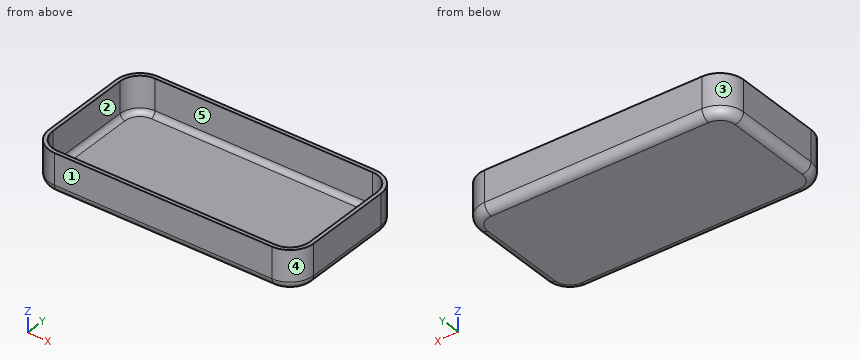
from build123d import *

# Parameters (mm, degrees)
F0_W     = 53.3
F0_H     = 27.3
F0_W_2   = 51.8
F0_H_2   = 25.8
F1_DEPTH = 0.75
F2_DEPTH = 8
F3_R     = 4
F4_R     = 4.75
F5_R     = 1
F6_R     = 1.75


with BuildPart() as f1:
    # F0 (on Top) → F1 (new body)
    with BuildSketch(Plane.XY):
        Rectangle(F0_W, F0_H)
        Rectangle(F0_W_2, F0_H_2, mode=Mode.SUBTRACT)
        Rectangle(F0_W_2, F0_H_2)
    extrude(amount=F1_DEPTH)

    # F0 (on Top) → F2 (join)
    with BuildSketch(Plane.XY):
        Rectangle(F0_W, F0_H)
        Rectangle(F0_W_2, F0_H_2, mode=Mode.SUBTRACT)
    extrude(amount=F2_DEPTH)

    # F3
    f3_edges = [f1.edges().sort_by_distance(p)[0] for p in [
        (-25.9, 12.9, 4.375),
        (25.9, 12.9, 4.375),
        (25.9, -12.9, 4.375),
        (-25.9, -12.9, 4.375),
    ]]
    fillet(f3_edges, radius=F3_R)

    # F4
    f4_edges = [f1.edges().sort_by_distance(p)[0] for p in [
        (26.65, 13.65, 4),
        (26.65, -13.65, 4),
        (-26.65, 13.65, 4),
        (-26.65, -13.65, 4),
    ]]
    fillet(f4_edges, radius=F4_R)

    # F5
    f5_edges = [f1.edges().sort_by_distance(p)[0] for p in [
        (0, 12.9, 0.75),
    ]]
    fillet(f5_edges, radius=F5_R)

    # F6
    f6_edges = [f1.edges().sort_by_distance(p)[0] for p in [
        (0, 13.65, 0),
    ]]
    fillet(f6_edges, radius=F6_R)


solid = f1.part
Can you work these out from the model? Positions are in its coordinate system, mm. Face numbers are marked on the shaded views. A direction names the side the tool comes from. Coordinates: 2 decimals unless noted, no trailing zeros. Loops run counter-clockwise (first coordinate to the right, second up) from the corner with the lowest first, then second, coordinate; pieces in that order, holes last. Notation, with made-up numbers: (81.25, 31) - (108.25, 31) arc R19 ccw to (108.25, 43) - close; hole circle Ø10 at (26, 84.25). An arc over 180 degrees is marked (long way). Answer as a JSON object with one key per item and string values. Group by question number.
Item 1: If we section it at B-B (y = -1.25): List the corners of the cut face in (x, z) for me, plus the area to 3 significant figures.
Item 2: If we section it at A-A (z = 5): List the corners of the cut face in (x, y) for me, plus the area to 3 significant figures.
Item 3: For pin 1 (1 mm diameter, centred on x = -6.5, y = -11, fed in from +Z), with a flat end and sliding along its axis, tell me the tip position at first contact or that it passes through.
Item 4: If we mould it in two halves opening along Y, with no side actions, what happens to the marked faces 3, 4 and 5? For each: released by +Y, released by -Y, zero draft, split by the parting line, or undercut.
Item 5: If we section it at C-C (x = -20): List the corners of the cut face in (y, z) for me, plus the area to 3 significant figures.
Item 6: If I drill on L1, parallel to X at y = -0.75, z = 3; L2, parallel to Y at x = 17, z = 7.25, over which ranges is the centre line in solid material (lowest first)? Write a range as from..to.
Item 7: On a 3-axis mill with a long thin cutter (end or side, diameter ignored), from which of +Z, -Z, +X, -X, +Y, -Y can I reach the whole of each face in a straight line? I mean the marked faces 1 and 2. Say none if no direction works.
Returned:
{
 "1": {"outline": "(-26.65, 1.75) arc R1.75 ccw to (-24.9, 0) - (24.9, 0) arc R1.75 ccw to (26.65, 1.75) - (26.65, 8) - (25.9, 8) - (25.9, 1.75) arc R1 cw to (24.9, 0.75) - (-24.9, 0.75) arc R1 cw to (-25.9, 1.75) - (-25.9, 8) - (-26.65, 8) - close", "area": "50.0 mm²"},
 "2": {"outline": "(-26.65, -8.9) arc R4.75 ccw to (-21.9, -13.65) - (21.9, -13.65) arc R4.75 ccw to (26.65, -8.9) - (26.65, 8.9) arc R4.75 ccw to (21.9, 13.65) - (-21.9, 13.65) arc R4.75 ccw to (-26.65, 8.9) - close; hole (-25.9, -8.9) arc R4 ccw to (-21.9, -12.9) - (21.9, -12.9) arc R4 ccw to (25.9, -8.9) - (25.9, 8.9) arc R4 ccw to (21.9, 12.9) - (-21.9, 12.9) arc R4 ccw to (-25.9, 8.9) - close", "area": "113 mm²"},
 "3": {"pin 1": "stops at z = 0.75"},
 "4": {"face 3": "released by +Y", "face 4": "released by -Y", "face 5": "undercut"},
 "5": {"outline": "(-13.65, 1.75) arc R1.75 ccw to (-11.9, 0) - (11.9, 0) arc R1.75 ccw to (13.65, 1.75) - (13.65, 8) - (12.9, 8) - (12.9, 1.75) arc R1 cw to (11.9, 0.75) - (-11.9, 0.75) arc R1 cw to (-12.9, 1.75) - (-12.9, 8) - (-13.65, 8) - close", "area": "30.5 mm²"},
 "6": {"L1": "x = -26.65..-25.9, 25.9..26.65", "L2": "y = -13.65..-12.9, 12.9..13.65"},
 "7": {"face 1": "+Z, -Z, +X, -X, -Y", "face 2": "+Z"}
}
